Autodesk Fusion 360 part; units mm, degrees
sketch "Sketch1" plane through (0, 0, 0) normal (0, 0, 1) x (1, 0, 0)
  line L0 (2.55, 1.55) -> (-2.55, -1.55) construction
  line L1 (2.55, 1.55) -> (-2.55, -1.55) construction
  line L2 (-2.55, 1.55) -> (-2.55, -1.55)
  circle A0 centre (0, 0) radius 4
  line L3 (-2.55, 1.55) -> (2.55, -1.55) construction
  line L4 (-2.55, -1.55) -> (2.55, -1.55)
  line L5 (2.55, 1.55) -> (-2.55, 1.55)
  line L6 (2.55, 1.55) -> (-2.55, -1.55) construction
  line L7 (-2.55, 1.55) -> (2.55, -1.55) construction
  line L8 (-2.55, 1.55) -> (2.55, -1.55) construction
  circle A1 centre (0, 0) radius 2.55
  line L9 (2.55, -1.55) -> (2.55, 1.55)
  line L10 (-10, 10) -> (10, 10)
  line L11 (10, 10) -> (10, -10)
  line L12 (10, -10) -> (-10, -10)
  line L13 (-10, -10) -> (-10, 10)
  circle A2 centre (-7, 7) radius 1.5
  line L14 (0, 10) -> (0, 7.5)
  circle A3 centre (7, 7) radius 1.5
  line L15 (-10, 0) -> (-8.5, 0)
  circle A4 centre (-7, -7) radius 1.5
  circle A5 centre (7, -7) radius 1.5
  dimension "d1" = 5.1
  dimension "d2" = 5.1
  dimension "d3" = 3.1
  dimension "d4" = 8
  dimension "d5" = 5.1
  dimension "d6" = 5.1
  dimension "d7" = 20
  dimension "d8" = 20
  dimension "d9" = 3
extrude "Extrude1" add sketch "Sketch1" along normal blind 10 contours L2 L5 A1 | L2 L4 A1 | L5 A1 | L4 A1 | L5 A1 L9 | L4 A1 L9 | A0 makes body 1
extrude "Extrude2" add sketch "Sketch1" against normal blind 3 separate body contours L10 L11 L12 L13 makes body 2
extrude "Extrude3" add sketch "Sketch1" against normal blind 3 contours L2 L5 A1 | L2 L4 A1 | L4 L5 A1 | L5 A1 | L4 A1 | L5 A1 L9 | L4 A1 L9 | A0 bodies 1 2
sketch "Sketch2" plane through (0, -1.55, 0) normal (0, 1, 0) x (-1, 0, 0)
  line L0 (-2.0248, 0) -> (2.0248, 0)
  line L1 (2.0248, 0) -> (2.0248, 10)
  line L2 (2.0248, 10) -> (-2.0248, 10)
  line L3 (-2.0248, 10) -> (-2.0248, 0)
  circle A0 centre (0.0464, 5) radius 1.5
  dimension "d18" = 3
extrude "Extrude4" cut sketch "Sketch2" against normal blind 3 contours A0 bodies 1
Work out the finished part from the listing and answer in its coordinate system (mm). A direction names the side the tool comes from. Give positions to 0.01 mm unless a question says otherwise; leave off trailing zeros. Order: outer loops, then holes, each group sorted by start corner. A loop starts at its lowest first (then second) coordinate and runs counter-clockwise, first axis right, second up. Notation, with made-up numbers: M 41.25,76.25 L 76.25,76.25 A34 ccw 76.25,112.25 Z; hole C -1.75,-9.75 d5. An arc over 180 degrees is marked long. Return JSON: item names as keys, results as strings.
1) A tool of negligible diameter and unlimited length cuts with its end or side. For faces 5 (the flat face through (-1.4, -1.55, 3.8)), 6 (the flat face through (0, -10, -1)), from which of +Z, -Z, +X, -X, +Y, -Y can it reach the whole face along a straight path? Write none if from no direction.
Resolved:
{"face 5": "+Z", "face 6": "+Z, -Z, +X, -X, -Y"}
2) For a pull along X with two mould halves and no side action, classify faces 1 (the cylindrical face through (0.149, -2.758, 6.487)), 2 (the flat face through (0, -2, 10)), 3 (the flat face through (-10, 0, -1)), 4 (the cylindrical face through (-0.867, 3.905, 4.93)) as +X half, -X half, draft (parallel to the pull), parting line (faces both ways), or undercut.
Resolved:
{"face 1": "undercut", "face 2": "draft", "face 3": "-X half", "face 4": "parting line"}
3) Section D-D, the plane y = -3.25 is taken. Write down the section's boundary in (x, z), plus the area to 3 significant figures.
Resolved:
{"outline": "M -10,-3 L 10,-3 L 10,0 L 2.33,0 L 2.33,10 L -2.33,10 L -2.33,0 L -10,0 Z; hole C -0.05,5 d3", "area": "99.6 mm^2"}
4) Section C-C, the plane z = -1.75 is taken. Write down the section's boundary in (x, y), plus the area to 3 significant figures.
Resolved:
{"outline": "M -10,-10 L 10,-10 L 10,10 L -10,10 Z; hole C -7,-7 d3; hole C -7,7 d3; hole C 7,-7 d3; hole C 7,7 d3", "area": "372 mm^2"}
5) Section A-A, the plane x = -7 is taken. Write down the section's boundary in (y, z), plus the area to 3 significant figures.
Resolved:
{"outline": "M -10,-3 L -8.5,-3 L -8.5,0 L -10,0 Z; M -5.5,-3 L 5.5,-3 L 5.5,0 L -5.5,0 Z; M 8.5,-3 L 10,-3 L 10,0 L 8.5,0 Z", "area": "42.0 mm^2"}
6) Each of these flat-tipped pins is pushed along its axis until it touches: pin 1 (5 mm diameter, centred on x = -7, y = 7, fed in from +Z); pin 2 (6 mm diameter, centred on x = 5.5, z = 7, fed in from +Y); pin 3 (1.8 mm diameter, centred on x = -0.05, z = 5, fed in from -Y). Where does it stop, or does it pass through?
Resolved:
{"pin 1": "z = 0", "pin 2": "y = 3.12", "pin 3": "y = 1.55"}
7) Straight lines are drawn through the part: line 1 along Y through (x, z) = (-7, -1); line 2 along Z through (x, y) = (1.5, -7); line 3 along Y through (x, z) = (6.25, -0.75). For each, find the intervals that lie inside material, in ascending order. Write a range as [from, to].
Resolved:
{"line 1": "[-10, -8.5], [-5.5, 5.5], [8.5, 10]", "line 2": "[-3, 0]", "line 3": "[-10, -8.3], [-5.7, 5.7], [8.3, 10]"}
